from build123d import *

# Parameters (mm, degrees)
F0_W      = 2.54
F0_H      = 1.27
F1_DEPTH  = 10.16
F2_R      = 0.254
F3_DEPTH  = 2.54
F4_R      = 0.3175
F5_DEPTH  = 2.54
F6_R      = 0.254
F7_DEPTH  = 2.54
F8_R      = 0.254
F9_DEPTH  = 2.54
F10_R     = 0.254
F11_DEPTH = 2.54


with BuildPart() as f1:
    # F0 (on Right) → F1 (new body)
    with BuildSketch(Plane.YZ):
        with Locations((-0.004628, 0.539757)):
            Rectangle(F0_W, F0_H)
        Polygon((1.265372, -0.095243), (-1.274628, -0.095243), (-0.384839, -2.635243), (0.377161, -2.635243), align=None)
    extrude(amount=F1_DEPTH)

    # F2 (on face) → F3 (cut)
    with BuildSketch(Plane(origin=(0, 0, -2.635243), x_dir=(1, 0, 0), z_dir=(0, 0, -1))):
        with Locations((1.27, 0)):
            Circle(F2_R)
    extrude(amount=-F3_DEPTH, mode=Mode.SUBTRACT)

    # F4 (on face) → F5 (join)
    with BuildSketch(Plane.XY.offset(1.174757)):
        with Locations((5.08, 0)):
            Circle(F4_R)
    extrude(amount=F5_DEPTH)

    # F6 (on face) → F7 (cut)
    with BuildSketch(Plane(origin=(0, 0, -2.635243), x_dir=(1, 0, 0), z_dir=(0, 0, -1))):
        with Locations((8.89, 0)):
            Circle(F6_R)
    extrude(amount=-F7_DEPTH, mode=Mode.SUBTRACT)

    # F8 (on face) → F9 (cut)
    with BuildSketch(Plane(origin=(0, 0, -2.635243), x_dir=(1, 0, 0), z_dir=(0, 0, -1))):
        with Locations((3.81, 0)):
            Circle(F8_R)
    extrude(amount=-F9_DEPTH, mode=Mode.SUBTRACT)

    # F10 (on face) → F11 (cut)
    with BuildSketch(Plane(origin=(0, 0, -2.635243), x_dir=(1, 0, 0), z_dir=(0, 0, -1))):
        with Locations((6.35, 0)):
            Circle(F10_R)
    extrude(amount=-F11_DEPTH, mode=Mode.SUBTRACT)


solid = f1.part
Can you work these out from the model? Positions are in its coordinate system, mm. Give positions to 0.01 mm unless a question says otherwise; leave off trailing zeros. Loops run counter-clockwise (first coordinate to the right, second up) from the corner with the lowest first, then second, coordinate; pieces in that order, holes last. Notation, with made-up numbers: (-37.75, 63) -> (-23.75, 63) arc R10 cw to (-23.75, 70) -> close; hole circle Ø4 at (41.25, 43.25). An arc over 180 degrees is marked (long way). Write item = value, one per line.
1) Suppose I cut it at D-D on x = 1.27. Write out the boundary of the cut face in (y, z), then the cut area to 3 significant figures.
Check result:
outline = (-1.27, -0.1) -> (-0.38, -2.64) -> (-0.25, -2.64) -> (-0.25, -0.1) -> (0.25, -0.1) -> (0.25, -2.64) -> (0.38, -2.64) -> (1.27, -0.1) -> (1.27, 1.17) -> (-1.27, 1.17) -> close
area = 6.13 mm2
2) Suppose I cut it at B-B on y = 0. Write out the boundary of the cut face in (x, z), then the cut area to 3 significant figures.
Check result:
outline = (0, -2.64) -> (1.02, -2.64) -> (1.02, -0.1) -> (1.52, -0.1) -> (1.52, -2.64) -> (3.56, -2.64) -> (3.56, -0.1) -> (4.06, -0.1) -> (4.06, -2.64) -> (6.1, -2.64) -> (6.1, -0.1) -> (6.6, -0.1) -> (6.6, -2.64) -> (8.64, -2.64) -> (8.64, -0.1) -> (9.14, -0.1) -> (9.14, -2.64) -> (10.16, -2.64) -> (10.16, 1.17) -> (5.4, 1.17) -> (5.4, 3.71) -> (4.76, 3.71) -> (4.76, 1.17) -> (0, 1.17) -> close
area = 35.2 mm2
3) Suppose I cut it at A-A on x = 7.75. Write out the boundary of the cut face in (y, z), then the cut area to 3 significant figures.
Check result:
outline = (-1.27, -0.1) -> (-0.38, -2.64) -> (0.38, -2.64) -> (1.27, -0.1) -> (1.27, 1.17) -> (-1.27, 1.17) -> close
area = 7.42 mm2
4) I need wall thicknesses on L1, parallel to X at y = 0, z = -1.65; L2, parallel to Z at x = 2.25, y = -0.2; L3, parallel to Y at x = 8.89, z = -1.1. Which ranges of each line are inside material? Lowest first, please. Write a range as from..to.
Check result:
L1 = 0..1.02, 1.52..3.56, 4.06..6.1, 6.6..8.64, 9.14..10.16
L2 = -2.64..1.17
L3 = -0.92..-0.25, 0.25..0.91
5) Suppose I cut it at C-C on z = -0.25. Write out the boundary of the cut face in (x, y).
Check result:
outline = (0, -1.22) -> (10.16, -1.22) -> (10.16, 1.21) -> (0, 1.21) -> close; hole circle Ø0.51 at (1.27, 0); hole circle Ø0.51 at (3.81, 0); hole circle Ø0.51 at (6.35, 0); hole circle Ø0.51 at (8.89, 0)
